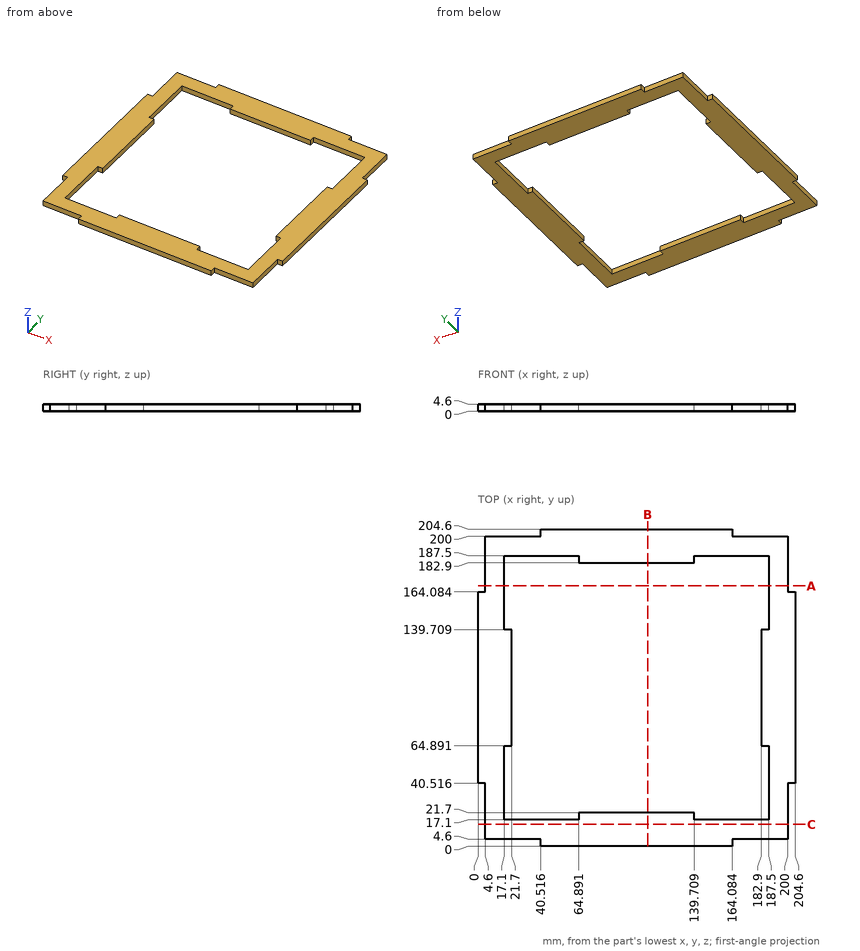
Can you work these out from the drawing? Everything is in mm from the part's minimum corner. Give positions to 0.01 mm unless a question says otherwise; leave off trailing zeros. Write each loop counter-clockwise with the first axis right and the second up, starting at its lowest first coordinate (ties: lowest second). Pieces come first, ordered by that corner, then holes. Notation, with made-up numbers: (69.25, 53.25) -> (104.25, 53.25) arc R17 ccw to (104.25, 61.25) -> close; hole circle Ø4 at (48.25, 77). An arc over 180 degrees is marked (long way). Write each question's results on one line, items separated by ' | '.
Item 1: Suppose I cut it at A-A on y = 168. Write out the boundary of the cut face in (x, z), plus the area to 3 significant figures.
Output:
outline: (4.6, 0) -> (17.1, 0) -> (17.1, 4.6) -> (4.6, 4.6) -> close; (187.5, 0) -> (200, 0) -> (200, 4.6) -> (187.5, 4.6) -> close | area: 115 mm^2
Item 2: Suppose I cut it at B-B on x = 109.5. Write out the boundary of the cut face in (y, z).
Output:
outline: (0, 0) -> (21.7, 0) -> (21.7, 4.6) -> (0, 4.6) -> close; (182.9, 0) -> (204.6, 0) -> (204.6, 4.6) -> (182.9, 4.6) -> close
Item 3: If I drill on L1, parallel to Y at x = 182, z = 3.1; L2, parallel to X at y = 155, z = 3.6, over which ranges is the centre line in solid material (lowest first)?
Output:
L1: y = 4.6 to 17.1, 187.5 to 200 | L2: x = 0 to 17.1, 187.5 to 204.6
Item 4: For pin 1 Ø1.4 at (x, z) = (171, 2) entering from -Y; pin 2 Ø1.4 at (x, z) = (202.5, 2) entering from -Y; pin 3 Ø2.5 at (x, z) = (31, 1.5) entering from +Y, each with a flat end and sliding along its axis, tell me the tip position at first contact or that it passes through.
Output:
pin 1: stops at y = 4.6 | pin 2: stops at y = 40.52 | pin 3: stops at y = 200
Item 5: Suppose I cut it at C-C on y = 14. Write out the boundary of the cut face in (x, z).
Output:
outline: (4.6, 0) -> (200, 0) -> (200, 4.6) -> (4.6, 4.6) -> close
